Part model, mm, in its own coordinate system. Face numbers are marked on the shaded views. A direction names the side the tool comes from. Coordinates: 2 decimals unless noted, no trailing zeros. Order: outer loops, then holes, each group sorted by start corner. A loop starts at its lowest first (then second) coordinate and runs counter-clockwise, first axis right, second up.
from build123d import *

# Parameters (mm, degrees)
EXTRUDE_1_DEPTH = 100
SKETCH_2_R      = 5
EXTRUDE_2_DEPTH = 2
SKETCH_3_W      = 80
SKETCH_3_H      = 80
EXTRUDE_3_DEPTH = 5
SKETCH_4_R      = 3
EXTRUDE_4_DEPTH = 8
SKETCH_5_W      = 60
SKETCH_5_H      = 40
EXTRUDE_5_DEPTH = 30
FILLET_1_R      = 2


with BuildPart() as part:
    # 草图1 → 凸台-拉伸1 (new body)
    with BuildSketch(Plane.XY):
        Polygon((0, 0), (-50, 0), (-50, 3), (50, 3), (50, 0), align=None)
    extrude(amount=-EXTRUDE_1_DEPTH)

    # 草图2 → 凸台-拉伸2 (add)
    with BuildSketch(Plane(origin=(0, 3, 0), x_dir=(1, 0, 0), z_dir=(0, 1, 0))):
        with Locations(Location((-30, 80, 0), (0, 0, 270))):
            Circle(SKETCH_2_R)
        with Locations(Location((30, 80, 0), (0, 0, 270))):
            Circle(SKETCH_2_R)
        with Locations(Location((-30, 20, 0), (0, 0, 270))):
            Circle(SKETCH_2_R)
        with Locations(Location((30, 20, 0), (0, 0, 270))):
            Circle(SKETCH_2_R)
    extrude(amount=EXTRUDE_2_DEPTH)

    # 草图3 → 凸台-拉伸3 (add)
    with BuildSketch(Plane(origin=(0, 5, 0), x_dir=(1, 0, 0), z_dir=(0, 1, 0))):
        with Locations((0, 50)):
            Rectangle(SKETCH_3_W, SKETCH_3_H)
    extrude(amount=EXTRUDE_3_DEPTH)

    # 草图4 → 凸台-拉伸4 (add)
    with BuildSketch(Plane(origin=(0, 10, 0), x_dir=(1, 0, 0), z_dir=(0, 1, 0))):
        with Locations(Location((-15, 65, 0), (0, 0, 90))):
            Circle(SKETCH_4_R)
        with Locations(Location((15, 65, 0), (0, 0, 90))):
            Circle(SKETCH_4_R)
        with Locations(Location((-15, 35, 0), (0, 0, 90))):
            Circle(SKETCH_4_R)
        with Locations(Location((15, 35, 0), (0, 0, 90))):
            Circle(SKETCH_4_R)
    extrude(amount=EXTRUDE_4_DEPTH)

    # 草图5 → 凸台-拉伸5 (add)
    with BuildSketch(Plane.XZ):
        with Locations((0, -50)):
            Rectangle(SKETCH_5_W, SKETCH_5_H)
    extrude(amount=EXTRUDE_5_DEPTH)

    # 圆角1
    fillet_1_edges = [part.edges().sort_by_distance(p)[0] for p in [
        (30, -15, -70),
        (30, -15, -30),
        (-30, -15, -30),
        (-30, -15, -70),
        (30, -30, -50),
        (0, -30, -30),
        (-30, -30, -50),
        (0, -30, -70),
    ]]
    fillet(fillet_1_edges, radius=FILLET_1_R)


solid = part.part
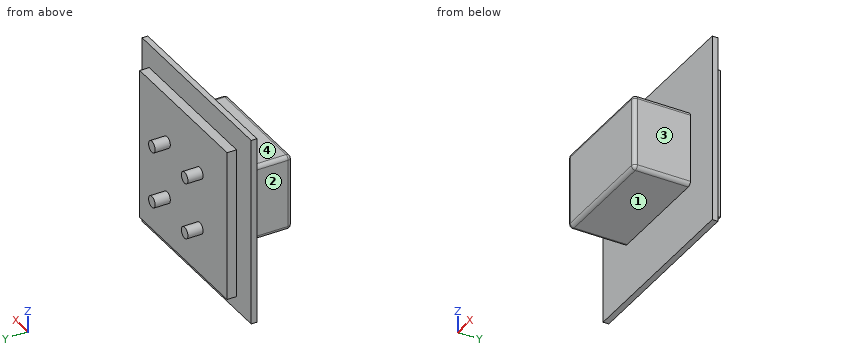
Q1. Pin check, flat tips, straight feed: pin 1 Ø8 at (x, y) = (-21, -20) entering from -Z; pin 2 Ø1 at (y, z) = (-9, -28) entering from +X; pin 3 Ø6 at (x, z) = (1.5, -21) entering from -Y; pin 4 Ø8 at (y, z) = (10, -68) entering from +X. Stop position of each tip, or through.
Results list:
pin 1: stops at z = -70
pin 2: passes through
pin 3: stops at y = 0
pin 4: stops at x = 40
Q2. Cut at D-D on x = -33. Write the cut outline in (y, z).
Results list:
outline: (0, -100) - (3, -100) - (3, -84) - (5, -84) - (5, -90) - (10, -90) - (10, -10) - (5, -10) - (5, -16) - (3, -16) - (3, 0) - (0, 0) - close; hole (3, -76) - (5, -76) - (5, -24) - (3, -24) - close
Q3. Cut at A-A on x = 9. Write the cut outline in (y, z).
Results list:
outline: (-30, -68) arc R2 ccw to (-28, -70) - (0, -70) - (0, -100) - (3, -100) - (3, 0) - (0, 0) - (0, -30) - (-28, -30) arc R2 ccw to (-30, -32) - close; (5, -90) - (10, -90) - (10, -10) - (5, -10) - close
Q4. Cut at B-B on z = -35. Write the cut outline in (x, y).
Results list:
outline: (-50, 0) - (-30, 0) - (-30, -28) arc R2 ccw to (-28, -30) - (28, -30) arc R2 ccw to (30, -28) - (30, 0) - (50, 0) - (50, 3) - (-50, 3) - close; (-40, 5) - (40, 5) - (40, 10) - (18, 10) - (18, 18) - (12, 18) - (12, 10) - (-12, 10) - (-12, 18) - (-18, 18) - (-18, 10) - (-40, 10) - close
Q5. Cut at C-C on z = -80. Write the cut outline in (x, y).
Results list:
outline: (-50, 0) - (50, 0) - (50, 3) - (35, 3) - (35, 5) - (40, 5) - (40, 10) - (-40, 10) - (-40, 5) - (-35, 5) - (-35, 3) - (-50, 3) - close; hole (-25, 3) - (25, 3) - (25, 5) - (-25, 5) - close
Q6. Which spindle directions (+Z, -Z, +X, -X, +Y, -Y) get a long thin tool onto all of the face, cutting with end or side? Do the marked faces 1, 2, 3 and 4. Say none if no direction does.
Results list:
face 1: -Z, +X, -X, -Y
face 2: +Z, -Z, -X, -Y
face 3: +Z, -Z, +X, -Y
face 4: +Z, +X, -X, -Y
Q7. Wall check: line 1 along Y through (x, z) = (-22, -81.5); line 2 along Y through (x, z) = (-18.5, -35.5); line 3 along Z through (x, y) = (8.5, -23). Give the ranges that are in metal, low to high.
Results list:
line 1: y = 0 to 3, 5 to 10
line 2: y = -30 to 3, 5 to 10
line 3: z = -70 to -30
